```python
from build123d import *

# Parameters (mm, degrees)
F1_DEPTH      = 19.05
F2_W          = 19.05
F2_H          = 25.4
F3_DEPTH      = 9.525
F3_DEPTH_BACK = 28.575


with BuildPart() as f1:
    # F0 (on Front) → F1 (new body)
    with BuildSketch(Plane.XZ):
        Polygon((-71.369838, 22.256227), (-71.369838, -41.243773), (55.630162, -41.243773), (55.630162, -9.493773), (-20.569838, -9.493773), (-45.969838, 22.256227), align=None)
    extrude(amount=F1_DEPTH)

    # F2 (on face) → F3 (join, two sides)
    with BuildSketch(Plane.XZ.offset(19.05)) as f3_sk:
        with Locations((-61.844838, -28.543773)):
            Rectangle(F2_W, F2_H)
    extrude(amount=F3_DEPTH)
    extrude(f3_sk.sketch, amount=-F3_DEPTH_BACK)


solid = f1.part
```
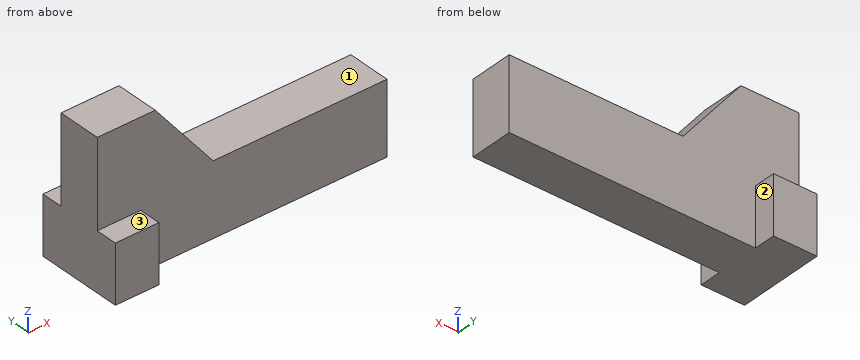
Check sheet for the modelled part. Datum: model origin and axes. Units: mm. Face numbers are marked on the shaded views. A direction names the side the tool comes from. Round coordinates to 2 decimals unless told otherwise and drop trailing zeros. Loops run counter-clockwise (first coordinate to the right, second up) from the corner with the lowest first, then second, coordinate; pieces in that order, holes last. Notation, with made-up numbers: (50, 39.25) -> (56, 39.25) arc R21 cw to (56, 45.25) -> close; hole circle Ø6 at (68, -23). An arc over 180 degrees is marked (long way). Answer in a Markdown table with one row per item.
Q1. Sectioned sample at D-D on y = -23. Enter the section's corners in (x, z), then the cut area to 3 significant figures.
Data:
| item | result |
|---|---|
| outline | (-71.37, -41.24) -> (-52.32, -41.24) -> (-52.32, -15.84) -> (-71.37, -15.84) -> close |
| area | 484 mm^2 |
Q2. Thickness scan on L1, parallel to Z at x = -4, y = -17.5; L2, parallel to Y at x = 3.5, z = -29; L3, parallel to X at y = -17, z = 16. Record the ranges inside material, lowest first.
Data:
| item | result |
|---|---|
| L1 | z = -41.24 to -9.49 |
| L2 | y = -19.05 to 0 |
| L3 | x = -71.37 to -40.96 |
Q3. Set-up check for the marked faces 1, 2 and 3: record each of +Z, -Z, +X, -X, +Y, -Y from which the full face is reachable in a straight line by a thin tool's end or side.
Data:
| item | result |
|---|---|
| face 1 | +Z, +X, +Y, -Y |
| face 2 | +Z, -Z, +X, +Y |
| face 3 | +Z, +X, -X, -Y |
Q4. Sectioned sample at B-B on y = -17.5. Enter the section's corners in (x, z).
Data:
| item | result |
|---|---|
| outline | (-71.37, -41.24) -> (55.63, -41.24) -> (55.63, -9.49) -> (-20.57, -9.49) -> (-45.97, 22.26) -> (-71.37, 22.26) -> close |
Q5. Sectioned sample at A-A on z = -28.5. Enter the section's corners in (x, y) (3 decimals), then the cut area to 3 significant figures.
Data:
| item | result |
|---|---|
| outline | (-71.37, -28.575) -> (-52.32, -28.575) -> (-52.32, -19.05) -> (55.63, -19.05) -> (55.63, 0) -> (-52.32, 0) -> (-52.32, 9.525) -> (-71.37, 9.525) -> close |
| area | 2,780 mm^2 |
Q6. Sectioned sample at C-C on x = -57. Enter the section's corners in (y, z) (3 decimals).
Data:
| item | result |
|---|---|
| outline | (-28.575, -41.244) -> (9.525, -41.244) -> (9.525, -15.844) -> (0, -15.844) -> (0, 22.256) -> (-19.05, 22.256) -> (-19.05, -15.844) -> (-28.575, -15.844) -> close |
Q7. Go/stop test with flat-tipped pins: P1, Ø2, axis at y = -20.5, z = 2, coming from the -X side; P2, Ø8, axis at x = -30.5, y = -4.5, coming from the +Z side; P3, Ø19, axis at x = 23.5, z = -10, coming from the +Y side; P4, Ø3, axis at x = -59, y = -26, coming from the +Z side. Record where each tip stops, or that it passes through.
Data:
| item | result |
|---|---|
| P1 | passes through |
| P2 | stops at z = 7.92 |
| P3 | stops at y = 0 |
| P4 | stops at z = -15.84 |
